```python
from build123d import *

# Parameters (mm, degrees)
SKETCH2_R           = 26
BOSS_EXTRUDE1_DEPTH = 5
FILLET3_R           = 25
SKETCH9_R           = 2
CUT_EXTRUDE2_DEPTH  = 4
FILLET5_R           = 5


with BuildPart() as part:
    # Sketch2 → Boss-Extrude1 (new, symmetric)
    with BuildSketch(Plane.XY):
        with BuildLine():
            Line((-35, 15), (-35, -30))
            Line((-35, -30), (35, -30))
            Line((35, -30), (35, 15))
            ThreePointArc((35, 15), (0, 35), (-35, 15))
        make_face()
        Circle(SKETCH2_R, mode=Mode.SUBTRACT)
    extrude(amount=BOSS_EXTRUDE1_DEPTH, both=True)

    # Fillet3
    fillet3_edges = [part.edges().sort_by_distance(p)[0] for p in [
        (35, 15, 0),
        (-35, 15, 0),
    ]]
    fillet(fillet3_edges, radius=FILLET3_R)

    # Sketch9 → Cut-Extrude2 (cut)
    with BuildSketch(Plane.XZ.offset(30)):
        with Locations(Location((-7.5, 0, 0), (0, 0, 270))):
            Circle(SKETCH9_R)
        with Locations(Location((7.5, 0, 0), (0, 0, 270))):
            Circle(SKETCH9_R)
    extrude(amount=-CUT_EXTRUDE2_DEPTH, mode=Mode.SUBTRACT)

    # Fillet5
    fillet5_edges = [part.edges().sort_by_distance(p)[0] for p in [
        (-35, -11.809571027, 5),
        (-35, -11.809571027, -5),
        (-32.638462845, 16.987459663, 5),
        (-32.638462845, 16.987459663, -5),
        (35, -11.809571027, -5),
        (35, -11.809571027, 5),
        (32.638462845, 16.987459663, 5),
        (32.638462845, 16.987459663, -5),
        (0, 35, 5),
        (0, 35, -5),
    ]]
    fillet(fillet5_edges, radius=FILLET5_R - 0.0001)  # a hair under: the kernel refuses the full size


solid = part.part
```
Model file for the job. Use its own axes, mm. A direction names the side the tool comes from. Coordinates: 2 decimals unless noted, no trailing zeros. Loops run counter-clockwise (first coordinate to the right, second up) from the corner with the lowest first, then second, coordinate; pieces in that order, holes last. Notation, with made-up numbers: M 33.25,-10.5 L 82.25,-10.5 A16 cw 82.25,13.5 Z; hole C 52.5,89.25 d10. An arc over 180 degrees is marked long. Use CSV: the item, a comma, the result in double quotes. Start each with the question number.
1. Tool access for faces 1 (the cylindrical face through (-5.517, -28.028, 0.26)), 2 (the cylindrical face through (34, -12, 3)): list every direction of +Z, -Z, +X, -X, +Y, -Y with a clear straight run to the whole face (end or side of a thin tool).
2. Band-saw the part on C-C, the plane z = 1. List the corners of the cut face in (x, y) (3 decimals).
3. Probe probe 1 along X at (y, z) = (-27.8, 0); probe 2 along Y at (x, z) = (0, -0.5); probe 3 along Y at (x, z) = (-14, 1.5). List the from-to ranges inside material, lowest first. Write a range as [from, to].
4. Flat gauge pins, fed straight in: pin 1 (2.5 mm diameter, centred on x = -7.5, z = 0, fed in from +Y); pin 2 (6 mm diameter, centred on y = 11.5, z = 0, fed in from +X); pin 3 (2.5 mm diameter, centred on x = 7.5, z = 0, fed in from -Y). Where does each tip first touch, or does it go through?
5. Two-plate mould, pull along X, no slides. Class faces 3 (the cylindrical face through (-34, -12, -3)), 4 (the flat face through (-0.4, -26.2, 5)), 5 (the cylindrical face through (-20.633, -15.821, -0.07)): pulls with the +X half, pulls with the -X half, needs draft (parallel to the pull), parting line crosses it, or undercut.
Entries:
1,face 1,"-Y"
1,face 2,"+Z, +X, +Y, -Y"
2,outline,"M -34.899,-30 L -9.232,-30 L -9.232,-26 L -5.768,-26 L -5.768,-30 L 5.768,-30 L 5.768,-26 L 9.232,-26 L 9.232,-30 L 34.899,-30 L 34.899,6.381 A24.899 ccw 25.935,25.513 A40.524 ccw -25.935,25.513 A24.899 ccw -34.899,6.381 Z; hole C 0,0 d52"
3,probe 1,"x = [-35, -9.5], [-5.5, 5.5], [9.5, 35]"
3,probe 2,"y = [-30, -26], [26, 34.97]"
3,probe 3,"y = [-30, -21.91], [21.91, 32.27]"
4,pin 1,"stops at y = 34.52"
4,pin 2,"stops at x = 34.91"
4,pin 3,"stops at y = -26"
5,face 3,"pulls with the -X half"
5,face 4,"needs draft"
5,face 5,"undercut"
